Autodesk Inventor part; units mm, degrees
ref_plane "GN300Klemmhebel_XY" through (0, 29.8, 20) normal (0, 0, 1) x (1, 0, 0)
ref_plane "GN300Klemmhebel_YZ" through (0, 29.8, 20) normal (1, 0, 0) x (0, 1, 0)
ref_plane "GN300Klemmhebel_ZX" through (0, 29.8, 20) normal (0, 1, 0) x (0, 0, 1)
sketch "Skizze_1" plane through (0, 0, 0) normal (0, 1, 0) x (-1, 0, 0)
  line L0 (20, -20) -> (20, 20)
  line L1 (20, 20) -> (-20, 20)
  line L2 (-20, 20) -> (-20, -20)
  line L3 (-20, -20) -> (20, -20)
extrude "Extrusion1" add sketch "Skizze_1" along normal blind 52
sketch "Skizze_2" plane through (0, 0, 0) normal (1, 0, 0) x (0, 1, 0)
  line L0 (55, 20) -> (46.5, 20)
  line L1 (46.5, 20) -> (46.5, 14)
  line L2 (46.5, 14) -> (8, 14)
  line L3 (8, 14) -> (8, -8)
  line L4 (8, -8) -> (46.5, -8)
  line L5 (46.5, -8) -> (46.5, -14)
  line L6 (46.5, -14) -> (8, -14)
  line L7 (8, -14) -> (8, -20)
  line L8 (8, -20) -> (55, -20)
  line L9 (55, -20) -> (55, 20)
extrude "Extrusion2" cut sketch "Skizze_2" along normal mid plane 42
sketch "Skizze_3" plane through (0, 0, 0) normal (0, 0, 1) x (1, 0, 0)
  line L0 (-20, 53) -> (-20, 8)
  line L1 (-20, 8) -> (-16.5, 8)
  line L2 (-16.5, 8) -> (-16.5, 30)
  arc A0 (16.5, 30) -> (-16.5, 30) centre (0, 30) ccw
  line L3 (16.5, 30) -> (16.5, 8)
  line L4 (16.5, 8) -> (20, 8)
  line L5 (20, 8) -> (20, 53)
  line L6 (20, 53) -> (-20, 53)
extrude "Extrusion3" cut sketch "Skizze_3" along normal mid plane 42
sketch "Sketch4" plane through (-20, 0, 20) normal (0, 0, 1) x (1, 0, 0)
  point P0 (20, 30)
hole "Hole1" at (0, 30, 20) direction (0, 0, -1) diameter 4.92 depth 39.8 countersink diameter 12 countersink angle 94.019
sketch "Sketch_1" plane through (0, 0, 0) normal (0, 1, 0) x (-1, 0, 0)
  line L0 (9.025, -10.45) -> (-9.025, -10.45)
  line L1 (-9.025, -10.45) -> (-9.025, -18.5)
  line L2 (-9.025, -18.5) -> (9.025, -18.5)
  line L3 (9.025, -18.5) -> (9.025, -10.45)
extrude "Extrusion4" cut sketch "Sketch_1" along normal blind 6.5
sketch "Sketch_2" plane through (0, 0, 0) normal (0, 1, 0) x (-1, 0, 0)
  line L0 (9.025, 10.45) -> (9.025, 18.5)
  line L1 (9.025, 18.5) -> (-9.025, 18.5)
  line L2 (-9.025, 18.5) -> (-9.025, 10.45)
  line L3 (-9.025, 10.45) -> (9.025, 10.45)
extrude "Extrusion5" cut sketch "Sketch_2" along normal blind 6.5
sketch "Sketch_3" plane through (0, 0, 0) normal (0, 1, 0) x (-1, 0, 0)
  line L0 (-10.45, 9.025) -> (-18.5, 9.025)
  line L1 (-18.5, 9.025) -> (-18.5, -9.025)
  line L2 (-18.5, -9.025) -> (-10.45, -9.025)
  line L3 (-10.45, -9.025) -> (-10.45, 9.025)
extrude "Extrusion6" cut sketch "Sketch_3" along normal blind 6.5
sketch "Sketch_4" plane through (0, 0, 0) normal (0, 1, 0) x (-1, 0, 0)
  line L0 (18.5, 9.025) -> (10.45, 9.025)
  line L1 (10.45, 9.025) -> (10.45, -9.025)
  line L2 (10.45, -9.025) -> (18.5, -9.025)
  line L3 (18.5, -9.025) -> (18.5, 9.025)
extrude "Extrusion7" cut sketch "Sketch_4" along normal blind 6.5
sketch "Sketch9" plane through (0, 0, 0) normal (0, -1, 0) x (1, 0, 0)
  point P0 (0, 0)
hole "Hole2" at (0, 0, 0) direction (0, 1, 0) diameter 8.5 depth 8
sketch "Sketch_5" plane through (0, 8, 0) normal (0, 1, 0) x (1, 0, 0)
  line L0 (-7.621, 0) -> (-3.8105, -6.6)
  line L1 (-3.8105, -6.6) -> (3.8105, -6.6)
  line L2 (3.8105, -6.6) -> (7.621, 0)
  line L3 (7.621, 0) -> (3.8105, 6.6)
  line L4 (3.8105, 6.6) -> (-3.8105, 6.6)
  line L5 (-3.8105, 6.6) -> (-7.621, 0)
extrude "Extrusion8" cut sketch "Sketch_5" against normal blind 4
ref_plane "GN300Klemmhebel_XY" through (0, 29.8, 20) normal (0, 0, 1) x (1, 0, 0)
ref_plane "GN300Klemmhebel_YZ" through (0, 29.8, 20) normal (1, 0, 0) x (0, 1, 0)
ref_plane "GN300Klemmhebel_ZX" through (0, 29.8, 20) normal (0, 1, 0) x (0, 0, 1)
ref_plane "GUS_4_41_XY" through (0, 29.8, 0) normal (0, 0, 1) x (1, 0, 0)
ref_plane "GUS_4_41_YZ" through (0, 29.8, 0) normal (1, 0, 0) x (0, 1, 0)
ref_plane "GUS_4_41_ZX" through (0, 29.8, 0) normal (0, 1, 0) x (0, 0, 1)
ref_plane "GUS_4_41_L_XY" through (0, 29.8, -20) normal (0, 0, 1) x (1, 0, 0)
ref_plane "GUS_4_41_L_YZ" through (0, 29.8, -20) normal (1, 0, 0) x (0, 1, 0)
ref_plane "GUS_4_41_L_ZX" through (0, 29.8, -20) normal (0, 1, 0) x (0, 0, 1)
ref_plane "GUS_4_41_R_XY" through (0, 29.8, 20) normal (0, 0, 1) x (1, 0, 0)
ref_plane "GUS_4_41_R_YZ" through (0, 29.8, 20) normal (1, 0, 0) x (0, 1, 0)
ref_plane "GUS_4_41_R_ZX" through (0, 29.8, 20) normal (0, 1, 0) x (0, 0, 1)
ref_plane "p0_XY" through (0, 0, 0) normal (0, 1, 0) x (1, 0, 0)
ref_plane "p0_YZ" through (0, 0, 0) normal (1, 0, 0) x (0, 0, -1)
ref_plane "p0_ZX" through (0, 0, 0) normal (0, 0, -1) x (0, 1, 0)
ref_plane "p1_XY" through (0, 0, -14.475) normal (0, 1, 0) x (1, 0, 0)
ref_plane "p1_YZ" through (0, 0, -14.475) normal (1, 0, 0) x (0, 0, -1)
ref_plane "p1_ZX" through (0, 0, -14.475) normal (0, 0, -1) x (0, 1, 0)
ref_plane "p2_XY" through (14.475, 0, 0) normal (0, 1, 0) x (1, 0, 0)
ref_plane "p2_YZ" through (14.475, 0, 0) normal (1, 0, 0) x (0, 0, -1)
ref_plane "p2_ZX" through (14.475, 0, 0) normal (0, 0, -1) x (0, 1, 0)
ref_plane "p3_XY" through (0, 0, 14.475) normal (0, 1, 0) x (1, 0, 0)
ref_plane "p3_YZ" through (0, 0, 14.475) normal (1, 0, 0) x (0, 0, -1)
ref_plane "p3_ZX" through (0, 0, 14.475) normal (0, 0, -1) x (0, 1, 0)
ref_plane "p4_XY" through (-14.475, 0, 0) normal (0, 1, 0) x (1, 0, 0)
ref_plane "p4_YZ" through (-14.475, 0, 0) normal (1, 0, 0) x (0, 0, -1)
ref_plane "p4_ZX" through (-14.475, 0, 0) normal (0, 0, -1) x (0, 1, 0)
ref_plane "ps_XY" through (0, 8, 0) normal (0, 1, 0) x (1, 0, 0)
ref_plane "ps_YZ" through (0, 8, 0) normal (1, 0, 0) x (0, 0, -1)
ref_plane "ps_ZX" through (0, 8, 0) normal (0, 0, -1) x (0, 1, 0)
chamfer "Chamfer1" distance 1.25 angle 45 4 edges at (-20, 4, -20) (-20, 4, 20) (20, 4, 20) (20, 4, -20)
properties part number "Robotunits GUS_4040 -90"
Can you work these out from the model? Positions are in its coordinate system, mm. A direction names the side the tool comes from. Round coordinates to 2 decimals unless told otherwise and drop trailing zeros. Loops run counter-clockwise (first coordinate to the right, second up) from the corner with the lowest first, then second, coordinate; pieces in that order, holes last.
Item 1: Suppose I cut it at C-C, the plane y = 40. Write out the boundary of the cut face in (x, z).
Item 2: Which directions (+Z, -Z, +X, -X, +Y, -Y) give clear straight access to the entire face, cutting with the end or side of a thin tool? Please do faces 1 (the flat face through (-5.689, 6.028, -3.346)), 2 (the flat face through (-16.5, 19, 17)), 3 (the flat face through (0, 6.5, -14)), 4 (the flat face through (20, 4, 0)).
Item 3: If we mould it in two halves opening along X, with no side actions, what happens to faces 5 (the flat face through (10.45, 3, 0)), 6 (the flat face through (0, 18, 20)), 7 (the flat face through (16.5, 19, -11))? For each: +X half, -X half, draft (parallel to the pull), parting line (faces both ways), or undercut.
Item 4: Will these pins go through, and if not, where does the flat tip stop? pin 1 Ø3 at (x, y) = (-2, 21) entering from -Z; pin 2 Ø6 at (x, z) = (15, -7) entering from +Y; pin 3 Ø6 at (x, z) = (-11, 10.5) entering from +Y; pin 4 Ø8 at (y, z) = (42, -1.5) entering from -X.
Item 5: Suppose I cut it at B-B, the plane z = 8. Write out the boundary of the cut face in (x, y).
Item 6: Suppose I cut it at D-D, the plane x = 0. State how many separate pieces and enclosed holes the cut face has, then the cut area to 3 significant figures.
Item 7: Please list where these lines run through material, in increasing order: L1, parallel to X at y = 1.45, z = 0; L2, parallel to Z at x = -12.5, y = 23.
Item 8: Suppose I cut it at A-A, the plane z = 16. Write out the boundary of the cut face in (x, y) (3 decimals).
Reported:
1. outline: (-13.12, -14) - (13.12, -14) - (13.12, -8) - (-13.12, -8) - close; (-13.12, 14) - (13.12, 14) - (13.12, 20) - (-13.12, 20) - close
2. face 1: +Y
2. face 2: +Z, -Z, -X, +Y
2. face 3: -Y
2. face 4: +Z, -Z, +X, +Y, -Y
3. face 5: undercut
3. face 6: draft
3. face 7: +X half
4. pin 1: stops at z = -14
4. pin 2: stops at y = 41.14
4. pin 3: stops at y = 8
4. pin 4: passes through
5. outline: (-20, 0) - (-18.5, 0) - (-18.5, 6.5) - (-10.45, 6.5) - (-10.45, 0) - (10.45, 0) - (10.45, 6.5) - (18.5, 6.5) - (18.5, 0) - (20, 0) - (20, 8) - (-20, 8) - close
6. separate pieces: 4
6. enclosed holes: 0
6. area: 520 mm2
7. L1: x = -20 to -18.5, -10.45 to -4.25, 4.25 to 10.45, 18.5 to 20
7. L2: z = -14 to -8, 14 to 20
8. outline: (-20, 0) - (-9.025, 0) - (-9.025, 6.5) - (9.025, 6.5) - (9.025, 0) - (20, 0) - (20, 8) - (16.5, 8) - (16.5, 30) arc R16.5 ccw to (-16.5, 30) - (-16.5, 8) - (-20, 8) - close; hole circle Ø4.92 at (0, 30)
